from build123d import *

# Parameters (mm, degrees)
EXTRUDE4_DEPTH     = 114.43
CUT_EXTRUDE1_DEPTH = 116.389135104
SKETCH3_R          = 1.55
CUT_EXTRUDE2_DEPTH = 1.65
CUT_EXTRUDE3_DEPTH = 3.4
SKETCH5_W          = 1.65
SKETCH5_H          = 3
CUT_EXTRUDE4_DEPTH = 1.65


with BuildPart() as part:
    # Sketch1 → Extrude4 (new body)
    with BuildSketch(Plane.XY):
        Polygon((0, 0), (11.24, 0), (11.24, 9.7), (0, 9.7), (0, 8.05), (9.59, 8.05), (9.59, 1.65), (0, 1.65), align=None)
    extrude(amount=EXTRUDE4_DEPTH)

    # Sketch2 → Cut-Extrude1 (cut, through all)
    with BuildSketch(Plane(origin=(11.24, 0, 0), x_dir=(0, 0, -1), z_dir=(1, 0, 0))):
        Polygon((-6.35, 1.65), (-1.65, 1.65), (-1.65, 3.3), (0, 3.3), (0, 0), (-6.35, 0), align=None)
        Polygon((0, 9.7), (-6.35, 9.7), (-6.35, 8.05), (-1.65, 8.05), (-1.65, 6.4), (0, 6.4), align=None)
    extrude(amount=-CUT_EXTRUDE1_DEPTH, mode=Mode.SUBTRACT)

    # Sketch3 → Cut-Extrude2 (cut)
    with BuildSketch(Plane(origin=(0, 9.7, 0), x_dir=(-1, 0, 0), z_dir=(0, 1, 0))):
        with Locations((-7.49, 19.05)):
            Circle(SKETCH3_R)
        with Locations((-7.49, 44.45)):
            Circle(SKETCH3_R)
        with Locations((-7.49, 69.85)):
            Circle(SKETCH3_R)
        with Locations((-7.49, 95.25)):
            Circle(SKETCH3_R)
        Polygon((0, 6.35), (0, 114.43), (-9.59, 114.43), (-9.59, 108.08), (-11.24, 108.08), (-11.24, 103.19), (-5.62, 103.19), (-5.62, 106.95), (-3.75, 106.95), (-3.75, 11.24), (-5.62, 11.24), (-5.62, 9.59), (-7.49, 9.59), (-7.49, 6.35), align=None)
    extrude(amount=-CUT_EXTRUDE2_DEPTH, mode=Mode.SUBTRACT)

    # Sketch4 → Cut-Extrude3 (cut)
    with BuildSketch(Plane.XZ):
        Polygon((7.49, 6.35), (7.49, 9.2), (5.62, 9.2), (5.62, 11.24), (0, 11.24), (0, 6.35), align=None)
        Polygon((0, 103.19), (9.59, 103.19), (9.59, 104.84), (6.35, 104.84), (6.35, 106.49), (9.59, 106.49), (9.59, 108.14), (11.24, 108.14), (11.24, 114.43), (0, 114.43), align=None)
    extrude(amount=-CUT_EXTRUDE3_DEPTH, mode=Mode.SUBTRACT)

    # Sketch5 → Cut-Extrude4 (cut)
    with BuildSketch(Plane(origin=(11.24, 0, 0), x_dir=(0, 0, -1), z_dir=(1, 0, 0))):
        with Locations((-113.605, 4.9)):
            Rectangle(SKETCH5_W, SKETCH5_H)
    extrude(amount=-CUT_EXTRUDE4_DEPTH, mode=Mode.SUBTRACT)


solid = part.part
Could you check a few things on this model? Use its own coordinates, in mm. A direction names the side the tool comes from. Give positions to 0.01 mm unless a question says otherwise; leave off trailing zeros. Order: outer loops, then holes, each group sorted by start corner. A loop starts at its lowest first (then second) coordinate and runs counter-clockwise, first axis right, second up. Notation, with made-up numbers: M -13,-1 L 16,-1 A31 ccw 16,32 Z; hole C 81,-22.75 d11. An arc over 180 degrees is marked long. One line per question, with ' | ' between items.
1. I want a section at B-B (y = 4.75). List the corners of the cut face in (x, z) for me, and give its area (3 significant figures).
Results:
outline: M 9.59,0 L 11.24,0 L 11.24,112.78 L 9.59,112.78 Z | area: 186 mm²
2. I'm going to push flat-ended pins straight in: pin 1 (0.8 mm diameter, centred on x = 10.5, y = 4.5, fed in from +Z); pin 2 (1.8 mm diameter, centred on x = 7.5, y = 9, fed in from +Z); pin 3 (1.3 mm diameter, centred on x = 4, y = 1, fed in from -Z); pin 4 (2 mm diameter, centred on x = 2, y = 8.5, fed in from -Z). Where does each tip first touch, or does it pass through?
Results:
pin 1: z = 112.78 | pin 2: z = 103.19 | pin 3: z = 11.24 | pin 4: through
3. For faces 1 (the face through (7.692, 8.887, 96.787)), 2 (the face through (7, 8.05, 56)), 3 (the face through (11.24, 5, 56)), which set-ups out of +Z, -Z, +X, -X, +Y, -Y let a thin tool reach every point of the face, with its end or its side?
Results:
face 1: +Y | face 2: +Z, -Z, -X | face 3: +Z, -Z, +X, +Y, -Y
4. I want a section at A-A (z = 95.25). List the corners of the cut face in (x, y) for me.
Results:
outline: M 0,0 L 11.24,0 L 11.24,9.7 L 9.04,9.7 L 9.04,8.05 L 9.59,8.05 L 9.59,1.65 L 0,1.65 Z; M 3.75,8.05 L 5.94,8.05 L 5.94,9.7 L 3.75,9.7 Z
5. If I drill on line 1 (X direction, y = 9.45, z = 69.85); line 2 (Y direction, x = 7.25, z = 47); line 3 (Y direction, x = 1.5, z = 70), over which ranges is the centre line in solid material (lowest first)?
Results:
line 1: 3.75 to 5.94, 9.04 to 11.24 | line 2: 0 to 1.65, 8.05 to 9.7 | line 3: 0 to 1.65
6. We'd pull the mould along Y, two halves only. Please class faces 4 (the face through (6, 0, 57)), 5 (the face through (5, 1.65, 54)), 6 (the face through (6.66, 8.89, 20.36)): +Y half, -Y half, draft (parallel to the pull), parting line (faces both ways), or undercut.
Results:
face 4: -Y half | face 5: undercut | face 6: draft
